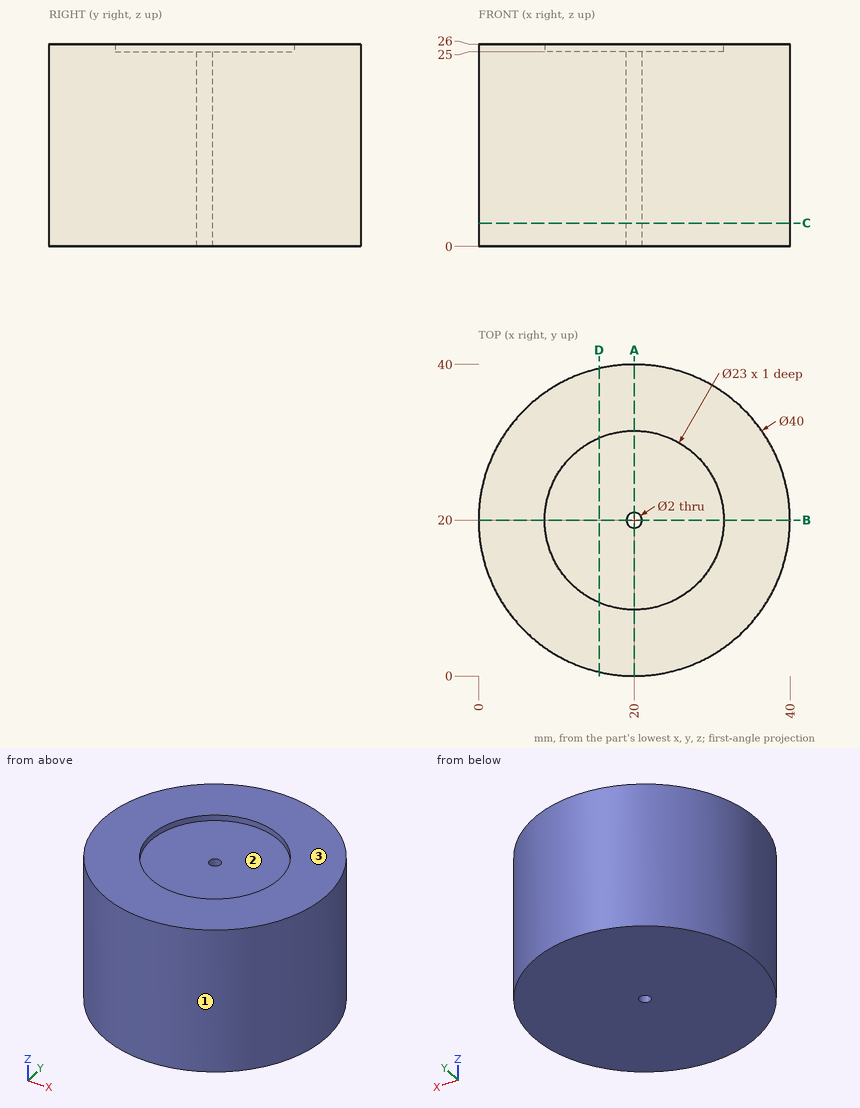
Answer from the drawing. Dimensions are ordinates in mm from the lowest x, y and z of the part. Coordinates: 2 decimals unless noted, no trailing zeros. Write each loop counter-clockwise with the first axis right and the second up, starting at its lowest first coordinate (ties: lowest second). Pieces come first, ordered by that corner, then holes. Notation, with made-up numbers: M 86.5,29 L 120.5,29 A28 ccw 120.5,66 Z; hole C 43,57.25 d7. An arc over 180 degrees is marked long. Use a Markdown table: item, result.
Q1. Determine the mould class of the marked faces 1, 2 and 3 for opening direction X: released by +X, released by -X, zero draft, split by the parting line, or undercut.
Answer block:
| item | result |
|---|---|
| face 1 | split by the parting line |
| face 2 | undercut |
| face 3 | zero draft |
Q2. The part is cut by section A-A, the plane x = 20. Write down the section's boundary in (y, z), then the cut area to 3 significant figures.
Answer block:
| item | result |
|---|---|
| outline | M 0,0 L 19,0 L 19,25 L 8.5,25 L 8.5,26 L 0,26 Z; M 21,0 L 40,0 L 40,26 L 31.5,26 L 31.5,25 L 21,25 Z |
| area | 967 mm2 |
Q3. Each of these flat-tipped pins is pushed along its axis until it touches: pin 1 Ø8 at (y, z) = (19, 16.5) entering from +X; pin 2 Ø12 at (y, z) = (28, 7.5) entering from +X; pin 3 Ø4 at (x, z) = (6.5, 11) entering from -Y; pin 4 Ø1 at (y, z) = (23, 5.5) entering from -X. Where does it stop, or does it pass through?
Answer block:
| item | result |
|---|---|
| pin 1 | stops at x = 40 |
| pin 2 | stops at x = 39.9 |
| pin 3 | stops at y = 3.64 |
| pin 4 | stops at x = 0.16 |
Q4. Straight lines are drawn through the part: L1, parallel to Y at x = 20, z = 25.55; L2, parallel to Y at x = 20, z = 9.75; L3, parallel to Z at x = 13.5, y = 15. For each, find the intervals that lie inside material, in ascending order. Write a range as [from, to].
Answer block:
| item | result |
|---|---|
| L1 | y = [0, 8.5], [31.5, 40] |
| L2 | y = [0, 19], [21, 40] |
| L3 | z = [0, 25] |
Q5. The part is cut by section C-C, the plane z = 3. Write down the section's boundary in (x, y), then the cut area to 3 significant figures.
Answer block:
| item | result |
|---|---|
| outline | C 20,20 d40; hole C 20,20 d2 |
| area | 1,250 mm2 |
Q6. The part is cut by section D-D, the plane x = 15.5. Write down the section's boundary in (y, z).
Answer block:
| item | result |
|---|---|
| outline | M 0.51,0 L 39.49,0 L 39.49,26 L 30.58,26 L 30.58,25 L 9.42,25 L 9.42,26 L 0.51,26 Z |
